```python
from build123d import *

# Parameters (mm, degrees)
BOSS_EXTRUDE1_DEPTH     = 8.5
BOSS_EXTRUDE2_DEPTH     = 3
BOSS_EXTRUDE3_DEPTH     = 3
SKETCH10_W              = 9.5
SKETCH10_H              = 5
BOSS_EXTRUDE4_DEPTH     = 15.78
SKETCH11_W              = 9.5
SKETCH11_H              = 2
BOSS_EXTRUDE5_DEPTH     = 40
BOSS_EXTRUDE6_DEPTH     = 6.09393
SKETCH14_R              = 1.8
CUT_EXTRUDE1_DEPTH      = 6.3
SKETCH15_W              = 51.153217575
SKETCH15_H              = 21.210560201
CUT_EXTRUDE3_DEPTH      = 19.78
SKETCH18_W              = 3
SKETCH18_H              = 3
BOSS_EXTRUDE7_DEPTH     = 8.5
FILLET1_R               = 0.75
BOSS_EXTRUDE8_DEPTH     = 1.5
FILLET2_R               = 0.75
BOSS_EXTRUDE9_DEPTH     = 17.5
SKETCH21_W              = 12.5
SKETCH21_H              = 6
CUT_EXTRUDE4_DEPTH      = 30.0000001
CUT_EXTRUDE4_DEPTH_BACK = 39.5000001


with BuildPart() as part:
    # Sketch3 → Revolve1 (revolve)
    with BuildSketch(Plane.XY):
        Polygon((-62.694264441, 11.733728816), (-64.884531744, 11.733728816), (-64.884531744, 5.639799249), (-60.884531744, 5.639799249), (-60.884531744, 6.650679103), (-62.884531744, 6.650679103), (-62.884531744, 10.250679103), (-60.884531744, 10.250679103), (-60.884531744, 11.733728816), align=None)
    revolve(axis=Axis((-49.744264441, 0, 0), (0, 1, 0)))

    # Sketch7 → Boss-Extrude1 (add)
    with BuildSketch(Plane(origin=(0, 11.733728816, 0), x_dir=(1, 0, 0), z_dir=(0, 1, 0))):
        with BuildLine():
            Line((-50.244264441, 15.132008921), (-50.244264441, 13.130751112))
            ThreePointArc((-50.244264441, 13.130751112), (-49.744264441, 13.140267302), (-49.244264441, 13.130751112))
            Line((-49.244264441, 13.130751112), (-49.244264441, 15.132008921))
            ThreePointArc((-49.244264441, 15.132008921), (-49.744264441, 15.140267302), (-50.244264441, 15.132008921))
        make_face()
    extrude(amount=BOSS_EXTRUDE1_DEPTH)

    # Sketch8 → Boss-Extrude2 (add)
    with BuildSketch(Plane(origin=(0, 20.233728816, 0), x_dir=(1, 0, 0), z_dir=(0, 1, 0))):
        with BuildLine():
            Line((-50.244264441, 15.132008921), (-50.244264441, 13.130751112))
            Line((-50.244264441, 13.130751112), (-50.244264441, -6.369248888))
            Line((-50.244264441, -6.369248888), (-49.244264441, -6.369248888))
            Line((-49.244264441, -6.369248888), (-49.244264441, 13.130751112))
            Line((-49.244264441, 13.130751112), (-49.244264441, 15.132008921))
            ThreePointArc((-49.244264441, 15.132008921), (-49.744264441, 15.140267302), (-50.244264441, 15.132008921))
        make_face()
    extrude(amount=-BOSS_EXTRUDE2_DEPTH)

    # Sketch9 → Boss-Extrude3 (add)
    with BuildSketch(Plane(origin=(0, 11.733728816, 0), x_dir=(1, 0, 0), z_dir=(0, 1, 0))):
        with BuildLine():
            Line((-54.494264441, 14.375854548), (-54.494264441, 39.375854548))
            Line((-54.494264441, 39.375854548), (-44.994264441, 39.375854548))
            Line((-44.994264441, 39.375854548), (-44.994264441, 14.375854548))
            ThreePointArc((-44.994264441, 14.375854548), (-47.092177082, 14.906177465), (-49.244264441, 15.132008921))
            ThreePointArc((-49.244264441, 15.132008921), (-49.744264441, 15.140267302), (-50.244264441, 15.132008921))
            ThreePointArc((-50.244264441, 15.132008921), (-52.3963518, 14.906177465), (-54.494264441, 14.375854548))
        make_face()
    extrude(amount=-BOSS_EXTRUDE3_DEPTH)

    # Sketch10 → Boss-Extrude4 (add)
    with BuildSketch(Plane.XZ.offset(-8.733728816)):
        with Locations((-49.744264441, -36.875854548)):
            Rectangle(SKETCH10_W, SKETCH10_H)
    extrude(amount=BOSS_EXTRUDE4_DEPTH)

    # Sketch11 → Boss-Extrude5 (add)
    with BuildSketch(Plane(origin=(0, 0, -39.375854548), x_dir=(-1, 0, 0), z_dir=(0, 0, -1))):
        with Locations((49.744264441, -6.046271184)):
            Rectangle(SKETCH11_W, SKETCH11_H)
    extrude(amount=BOSS_EXTRUDE5_DEPTH)

    # Sketch13 → Boss-Extrude6 (add)
    with BuildSketch(Plane(origin=(0, 11.733728816, 0), x_dir=(1, 0, 0), z_dir=(0, 1, 0))):
        with BuildLine():
            Line((-28.603997139, 3.15), (-34.935307895, 3.15))
            ThreePointArc((-34.935307895, 3.15), (-34.603997139, 0), (-34.935307895, -3.15))
            Line((-34.935307895, -3.15), (-28.603997139, -3.15))
            Line((-28.603997139, -3.15), (-28.603997139, 3.15))
        make_face()
        with BuildLine():
            Line((-70.884531744, 3.15), (-70.884531744, -3.15))
            Line((-70.884531744, -3.15), (-64.553220987, -3.15))
            ThreePointArc((-64.553220987, -3.15), (-64.884531744, 0), (-64.553220987, 3.15))
            Line((-64.553220987, 3.15), (-70.884531744, 3.15))
        make_face()
    extrude(amount=-BOSS_EXTRUDE6_DEPTH)

    # Sketch14 → Cut-Extrude1 (cut)
    with BuildSketch(Plane.XY.offset(3.15)):
        with Locations((-31.769652517, 8.686764033)):
            Circle(SKETCH14_R)
        with Locations((-67.718876365, 8.686764033)):
            Circle(SKETCH14_R)
    extrude(amount=-CUT_EXTRUDE1_DEPTH, mode=Mode.SUBTRACT)

    # Sketch15 → Cut-Extrude3 (cut, through all)
    with BuildSketch(Plane(origin=(0, 11.733728816, 0), x_dir=(1, 0, 0), z_dir=(0, 1, 0))):
        with Locations((-49.018725857, -10.6052801)):
            Rectangle(SKETCH15_W, SKETCH15_H)
    extrude(amount=-CUT_EXTRUDE3_DEPTH, mode=Mode.SUBTRACT)

    # Sketch18 → Boss-Extrude7 (add)
    with BuildSketch(Plane(origin=(0, 11.733728816, 0), x_dir=(1, 0, 0), z_dir=(0, 1, 0))):
        with Locations((-49.744264441, 13.632008921)):
            Rectangle(SKETCH18_W, SKETCH18_H)
    extrude(amount=BOSS_EXTRUDE7_DEPTH)

    # Fillet1
    fillet1_edges = [part.edges().sort_by_distance(p)[0] for p in [
        (-50.744264441, 11.733728816, -15.132008921),
        (-48.744264441, 11.733728816, -15.132008921),
        (-49.744264441, 11.733728816, -12.132008921),
        (-48.244264441, 11.733728816, -13.632008921),
        (-51.244264441, 11.733728816, -13.632008921),
        (-49.744264441, 11.733728816, -15.140267302),
    ]]
    fillet(fillet1_edges, radius=FILLET1_R)

    # Sketch19 → Boss-Extrude8 (add)
    with BuildSketch(Plane(origin=(0, 20.233728816, 0), x_dir=(1, 0, 0), z_dir=(0, 1, 0))):
        with BuildLine():
            Line((-50.244264441, 15.132008921), (-51.244264441, 15.132008921))
            Line((-51.244264441, 15.132008921), (-51.244264441, 12.132008921))
            Line((-51.244264441, 12.132008921), (-50.244264441, 12.132008921))
            Line((-50.244264441, 12.132008921), (-50.244264441, -6.369248888))
            Line((-50.244264441, -6.369248888), (-49.244264441, -6.369248888))
            Line((-49.244264441, -6.369248888), (-49.244264441, 12.132008921))
            Line((-49.244264441, 12.132008921), (-48.244264441, 12.132008921))
            Line((-48.244264441, 12.132008921), (-48.244264441, 15.132008921))
            Line((-48.244264441, 15.132008921), (-49.244264441, 15.132008921))
            ThreePointArc((-49.244264441, 15.132008921), (-49.744264441, 15.140267302), (-50.244264441, 15.132008921))
        make_face()
    extrude(amount=BOSS_EXTRUDE8_DEPTH)

    # Fillet2
    fillet2_edges = [part.edges().sort_by_distance(p)[0] for p in [
        (-50.244264441, 19.483728816, -12.132008921),
        (-49.244264441, 19.483728816, -12.132008921),
    ]]
    fillet(fillet2_edges, radius=FILLET2_R)

    # Sketch20 → Boss-Extrude9 (add)
    with BuildSketch(Plane(origin=(0, 0, -79.375854548), x_dir=(-1, 0, 0), z_dir=(0, 0, -1))):
        with BuildLine():
            Line((15.994264441, -27.546271184), (17.994264441, -27.546271184))
            add(Edge.make_bspline(
                [(17.994264441, -27.546271184), (25.87775722, -9.327062953), (44.994264441, -7.046271184)],
                knots=[0, 0, 0, 0.444959485, 0.444959485, 0.444959485], degree=2))
            Line((44.994264441, -7.046271184), (54.494264441, -7.046271184))
            add(Edge.make_bspline(
                [(54.494264441, -7.046271184), (73.610771663, -9.327062953), (81.494264441, -27.546271184)],
                knots=[0.555040515, 0.555040515, 0.555040515, 1, 1, 1], degree=2))
            Line((81.494264441, -27.546271184), (83.494264441, -27.546271184))
            add(Edge.make_bspline(
                [(54.494264441, -5.046271184), (75.013161261, -7.38841158), (83.494264441, -27.546271184)],
                knots=[0.551684944, 0.551684944, 0.551684944, 1, 1, 1], degree=2))
            Line((54.494264441, -5.046271184), (44.994264441, -5.046271184))
            add(Edge.make_bspline(
                [(15.994264441, -27.546271184), (24.475367621, -7.38841158), (44.994264441, -5.046271184)],
                knots=[0, 0, 0, 0.448315056, 0.448315056, 0.448315056], degree=2))
        make_face()
    extrude(amount=-BOSS_EXTRUDE9_DEPTH)

    # Sketch21 → Cut-Extrude4 (cut, two sides)
    with BuildSketch(Plane(origin=(-44.994264441, 0, 0), x_dir=(0, 0, -1), z_dir=(1, 0, 0))) as cut_extrude4_sk:
        with Locations((70.625854548, -22.546271184)):
            Rectangle(SKETCH21_W, SKETCH21_H)
    extrude(amount=CUT_EXTRUDE4_DEPTH, mode=Mode.SUBTRACT)
    extrude(cut_extrude4_sk.sketch, amount=-CUT_EXTRUDE4_DEPTH_BACK, mode=Mode.SUBTRACT)


solid = part.part
```
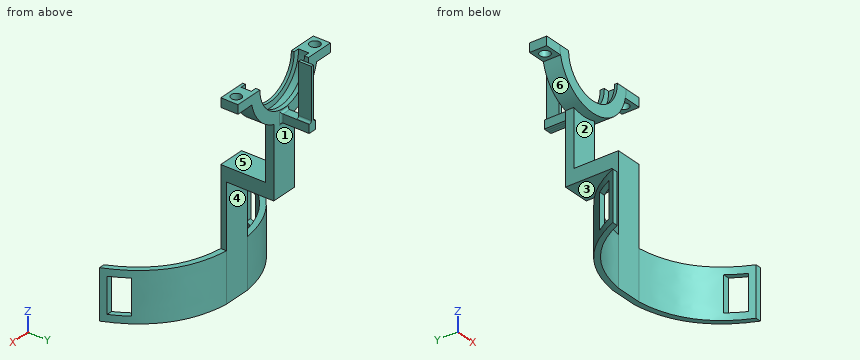
Input: part model. Units: mm. Frame: model coordinates. Face numbers are marked on the shaded views. A direction names the side the tool comes from. Give positions to 0.01 mm unless a question says otherwise; leave off trailing zeros. Write each loop counter-clockwise with the first axis right and the second up, starting at its lowest first coordinate (ties: lowest second). Pieces come first, ordered by that corner, then holes. Notation, with made-up numbers: (-30, 36) - (-16, 36) arc R27 ccw to (-16, 58) - close; hole circle Ø2 at (85.5, 76). An arc over 180 degrees is marked (long way). Write item = value, one per line. Start each with the question number.
1. Section query A-A, the plane z = -19.5. Output: boundary loops of the cut face in (x, y).
2. Ray query, L1, parallel to Y at x = -54.5, z = -64.5; L2, parallel to Z at x = -52.5, y = 7; L3, parallel to Y at x = -40.5, z = -10.5. Return the intervals inside material, ascending.
3. Access query for the marked faces 4, 5 and 6. Directions: +Z, -Z, +X, -X, +Y, -Y. A direction counts if a zero-diameter tool reaches every point of the face in a straight line with its end or side. Return the directions, or none.
4. Mould query, pull axis Z, two halves, no side actions, for the marked faces 1, 2 and 3. Classes: released by +Z, released by -Z, zero draft, split by the parting line, or undercut.
5. First-contact query: pin 1 Ø2.5 at (y, z) = (9.5, -2) entering from +X; pin 2 Ø18 at (x, y) = (-63, -18.5) entering from +Z; pin 3 Ø1 at (x, z) = (-18, -73.5) entering from +Y. Flat tips, straight axial feed; report the tip coordinate or a pass-through.
Check sheet entries:
q1.outline = (-54.49, 8.73) - (-44.99, 8.73) - (-44.99, 11.73) - (-54.49, 11.73) - close
q2.L1 = -7.05 to -5.05
q2.L2 = -39.38 to -34.38, -14.89 to -12.85
q2.L3 = 5.64 to 11.73
q3.face_4 = -Z, +X, -X, +Y
q3.face_5 = +X, -X, -Y
q3.face_6 = -Y
q4.face_1 = zero draft
q4.face_2 = undercut
q4.face_3 = released by -Z
q5.pin_1 = -28.6
q5.pin_2 = -61.88
q5.pin_3 = -25.55
